from build123d import *

# Parameters (mm, degrees)
SKETCH1_R           = 86.9315
BOSS_EXTRUDE1_DEPTH = 2.54
SKETCH2_W           = 50.8
SKETCH2_H           = 50.8
BOSS_EXTRUDE2_DEPTH = 304.8
SKETCH3_W           = 106.68
SKETCH3_H           = 106.68
BOSS_EXTRUDE4_DEPTH = 31.75
SKETCH4_W           = 101.6
SKETCH4_H           = 101.6
CUT_EXTRUDE1_DEPTH  = 29.21
SKETCH6_R           = 9.525
CUT_EXTRUDE3_DEPTH  = 29.21


with BuildPart() as part:
    # Sketch1 → Boss-Extrude1 (new body)
    with BuildSketch(Plane(origin=(0, 0, 0), x_dir=(1, 0, 0), z_dir=(0, 1, 0))):
        with Locations(Location((0, 0, 0), (0, 0, 270))):
            Circle(SKETCH1_R)
    extrude(amount=BOSS_EXTRUDE1_DEPTH)

    # Sketch2 → Boss-Extrude2 (add)
    with BuildSketch(Plane(origin=(0, 2.54, 0), x_dir=(1, 0, 0), z_dir=(0, 1, 0))):
        Rectangle(SKETCH2_W, SKETCH2_H)
    extrude(amount=BOSS_EXTRUDE2_DEPTH)

    # Sketch3 → Boss-Extrude4 (add)
    with BuildSketch(Plane(origin=(0, 307.34, 0), x_dir=(1, 0, 0), z_dir=(0, 1, 0))):
        Rectangle(SKETCH3_W, SKETCH3_H)
    extrude(amount=BOSS_EXTRUDE4_DEPTH)

    # Sketch4 → Cut-Extrude1 (cut)
    with BuildSketch(Plane(origin=(0, 339.09, 0), x_dir=(1, 0, 0), z_dir=(0, 1, 0))):
        Rectangle(SKETCH4_W, SKETCH4_H)
    extrude(amount=-CUT_EXTRUDE1_DEPTH, mode=Mode.SUBTRACT)

    # Sketch6 → Cut-Extrude3 (cut)
    with BuildSketch(Plane(origin=(0, 2.54, 0), x_dir=(1, 0, 0), z_dir=(0, 1, 0))):
        with Locations(Location((0, 69.50075, 0), (0, 0, 270))):
            Circle(SKETCH6_R)
        with Locations(Location((69.50075, 0, 0), (0, 0, 270))):
            Circle(SKETCH6_R)
        with Locations(Location((0, -69.50075, 0), (0, 0, 270))):
            Circle(SKETCH6_R)
        with Locations(Location((-69.50075, 0, 0), (0, 0, 270))):
            Circle(SKETCH6_R)
    extrude(amount=-CUT_EXTRUDE3_DEPTH, mode=Mode.SUBTRACT)


solid = part.part
Input: part model. Units: mm. Frame: model coordinates. A direction names the side the tool comes from. Give positions to 0.01 mm unless a question says otherwise; leave off trailing zeros. Loops run counter-clockwise (first coordinate to the right, second up) from the corner with the lowest first, then second, coordinate; pieces in that order, holes last. Notation, with made-up numbers: M -12,21 L 46,21 A10 cw 46,38 Z; hole C 23,19 d8. An arc over 180 degrees is marked long. Use one line per item in the form item = value.
1. First-contact query: pin 1 (23.5 mm diameter, centred on y = 321.5, z = -19, fed in from -X); pin 2 (9.5 mm diameter, centred on y = 320, z = -12, fed in from +X); pin 3 (8 mm diameter, centred on y = 234, z = -21, fed in from -X); pin 4 (15 mm diameter, centred on x = 0, z = 69.5, fed in from -Y). Flat tips, straight axial feed; report the tip coordinate or a pass-through.
Numbers:
pin_1 = -53.34
pin_2 = 53.34
pin_3 = -25.4
pin_4 = through
2. Reachability of faces 1 (the face through (-36, 307.34, -1)), 2 (the face through (-53.34, 323, 1)), 3 (the face through (-1, 325, 50.8)), 4 (the face through (0, 153, 25.4)) from +Z, -Z, +X, -X, +Y, -Y: full face, straight path, thin tool, end or side. Return the list, or none.
Numbers:
face_1 = none
face_2 = +Z, -Z, -X, +Y
face_3 = +Y
face_4 = +Z, +X, -X
3. Section query D-D, the plane x = 38. Return the cut outline in (y, z), and give its area (3 significant figures).
Numbers:
outline = M 0,-78.19 L 2.54,-78.19 L 2.54,78.19 L 0,78.19 Z; M 307.34,-53.34 L 339.09,-53.34 L 339.09,-50.8 L 309.88,-50.8 L 309.88,50.8 L 339.09,50.8 L 339.09,53.34 L 307.34,53.34 Z
area = 817 mm²
4. Line query: L1, parallel to Y at x = 49.5, z = -49.5; L2, parallel to Y at x = 53, z = 31; L3, parallel to X at y = 323.5, z = -51. Output: solid intervals per line, ascending.
Numbers:
L1 = 0 to 2.54, 307.34 to 309.88
L2 = 0 to 2.54, 307.34 to 339.09
L3 = -53.34 to 53.34
5. Pull-direction query (Y, two-part tool) for faces 5 (the face through (25.4, 153, 0)), 6 (the face through (1, 0, -1)), 7 (the face through (77.532, 1.288, 5.121)), 8 (the face through (-25.4, 153, 0)); classes: released by +Y, released by -Y, zero draft, split by the parting line, or undercut.
Numbers:
face_5 = undercut
face_6 = released by -Y
face_7 = zero draft
face_8 = undercut
6. Section query C-C, the plane z = -65.5. Return the cut outline in (x, y).
Numbers:
outline = M -57.16,0 L -8.64,0 L -8.64,2.54 L -57.16,2.54 Z; M 8.64,0 L 57.16,0 L 57.16,2.54 L 8.64,2.54 Z
7. Section query A-A, the plane x = 0. Return the cut outline in (y, z).
Numbers:
outline = M 0,-86.93 L 2.54,-86.93 L 2.54,-79.03 L 0,-79.03 Z; M 0,-59.98 L 2.54,-59.98 L 2.54,-25.4 L 307.34,-25.4 L 307.34,-53.34 L 339.09,-53.34 L 339.09,-50.8 L 309.88,-50.8 L 309.88,50.8 L 339.09,50.8 L 339.09,53.34 L 307.34,53.34 L 307.34,25.4 L 2.54,25.4 L 2.54,59.98 L 0,59.98 Z; M 0,79.03 L 2.54,79.03 L 2.54,86.93 L 0,86.93 Z
8. Section query B-B, the plane z = 0. Return the cut outline in (x, y).
Numbers:
outline = M -86.93,0 L -79.03,0 L -79.03,2.54 L -86.93,2.54 Z; M -59.98,0 L 59.98,0 L 59.98,2.54 L 25.4,2.54 L 25.4,307.34 L 53.34,307.34 L 53.34,339.09 L 50.8,339.09 L 50.8,309.88 L -50.8,309.88 L -50.8,339.09 L -53.34,339.09 L -53.34,307.34 L -25.4,307.34 L -25.4,2.54 L -59.98,2.54 Z; M 79.03,0 L 86.93,0 L 86.93,2.54 L 79.03,2.54 Z
